Autodesk Fusion 360 part; units mm, degrees
sketch "Sketch1" plane through (0, 0, 0) normal (0, 1, 0) x (1, 0, 0)
  circle A0 centre (0, 0) radius 20
  line L0 (-13.9601, 46.4878) -> (-27.9202, 10.9756)
  arc A1 (-27.9202, 10.9756) -> (27.9202, 10.9756) centre (0, 0) ccw
  line L1 (27.9202, 10.9756) -> (13.9601, 46.4878)
  arc A2 (13.9601, 46.4878) -> (-13.9601, 46.4878) centre (0, 41) ccw
  circle A3 centre (0, 41) radius 5
  point P0 (0, -30)
  point P1 (0, 56)
  dimension "d1" = 40
  dimension "d2" = 30
  dimension "d3" = 41
  dimension "d4" = 15
  dimension "d8" = 10
  dimension "d9" = 86
extrude "Extrude1" add sketch "Sketch1" along normal blind 20
chamfer "Chamfer1" distance 1 angle 45 12 edges at (0, 20, -56) (-20.9401, 20, -28.7317) (0, 20, 30) (20.9401, 20, -28.7317) (0, 0, -56) (-20.9401, 0, -28.7317) (0, 0, 30) (20.9401, 0, -28.7317) (-18.6465, 20, -7.2323) (-18.6465, 0, -7.2323) (-4.6616, 20, -42.8081) (-4.6616, 0, -42.8081)
Design review of the part built by this model. Coordinates are the model's own, in mm. Round coordinates to 2 decimals unless told otherwise and drop trailing zeros. Loops run counter-clockwise (first coordinate to the right, second up) from the corner with the lowest first, then second, coordinate; pieces in that order, holes last. Notation, with made-up numbers: (83.25, 81.25) - (136.25, 81.25) arc R5 ccw to (136.25, 88.25) - close; hole circle Ø4 at (5, 9). An arc over 180 degrees is marked (long way). One line per question, with ' | ' between items.
1. We need section C-C, the plane y = 3.25. State the section outline as (x, z) points, and give its area (3 significant figures).
Results are:
outline: (-27.92, -10.98) - (-13.96, -46.49) arc R15 ccw to (13.96, -46.49) - (27.92, -10.98) arc R30 ccw (long way) to start; hole circle Ø40 at (0, 0); hole circle Ø10 at (0, -41) | area: 2,400 mm²
2. Clearance check with flat-ended pins moving along their axes: P1, Ø8, axis at y = 7.5, z = -37, coming from the +X side; P2, Ø5, axis at x = 18, y = 12.5, coming from the +Z side; P3, Ø10, axis at y = 16.5, z = 1, coming from the +X side; P4, Ø1.5, axis at x = -8.5, z = 16, coming from the +Y side. State where each tip first meets the part, or that it passes through.
Results are:
P1: stops at x = 19.26 | P2: stops at z = 25.69 | P3: stops at x = 30 | P4: passes through
3. We need section D-D, the plane z = -41. State the section outline as (x, y) points, and give its area (3 significant figures).
Results are:
outline: (-16.12, 1) - (-15.04, 0) - (-6, 0) - (-5, 1) - (-5, 19) - (-6, 20) - (-15.04, 20) - (-16.12, 19) - close; (5, 1) - (6, 0) - (15.04, 0) - (16.12, 1) - (16.12, 19) - (15.04, 20) - (6, 20) - (5, 19) - close | area: 441 mm²
4. For L1, parallel to Z at x = 1, y = 1.25; L2, parallel to X at y = 11, z = 0.5; L3, parallel to Z at x = 7.5, y = 2.75, list the stretches that pass through material, from the lowest coordinate up. Write a range as [from, to].
Results are:
L1: z = [-55.97, -45.9], [-36.1, -19.97], [19.97, 29.98] | L2: x = [-30, -19.99], [19.99, 30] | L3: z = [-53.99, -18.54], [18.54, 29.05]
5. Draft analysis for pull direction Z (two halves, no side actions). For faces 1 (the face through (0, 10, -56)), 2 (the face through (-0.79, 0.17, 29.16)), 3 (the face through (-4.336, 9.874, -19.524)), state which applies: released by +Z, released by -Z, zero draft, split by the parting line, or undercut.
Results are:
face 1: released by -Z | face 2: split by the parting line | face 3: undercut
6. We need section A-A, the plane x = 0. State the section outline as (y, z) points, and give its area (3 significant figures).
Results are:
outline: (0, -55) - (1, -56) - (19, -56) - (20, -55) - (20, -47) - (19, -46) - (1, -46) - (0, -47) - close; (0, -35) - (1, -36) - (19, -36) - (20, -35) - (20, -21) - (19, -20) - (1, -20) - (0, -21) - close; (0, 21) - (1, 20) - (19, 20) - (20, 21) - (20, 29) - (19, 30) - (1, 30) - (0, 29) - close | area: 714 mm²
7. We need section B-B, the plane z = 0. State the section outline as (x, y) points, and give its area (3 significant figures).
Results are:
outline: (-30, 1) - (-29, 0) - (-21, 0) - (-20, 1) - (-20, 19) - (-21, 20) - (-29, 20) - (-30, 19) - close; (20, 1) - (21, 0) - (29, 0) - (30, 1) - (30, 19) - (29, 20) - (21, 20) - (20, 19) - close | area: 396 mm²
